Verification items for the finished model (mm, model axes). A direction names the side the tool comes from. Round coordinates to 2 decimals unless told otherwise and drop trailing zeros. Order: outer loops, then holes, each group sorted by start corner. A loop starts at its lowest first (then second) coordinate and runs counter-clockwise, first axis right, second up. Notation, with made-up numbers: (4.5, -17) -> (23.5, -17) arc R23 ccw to (23.5, 5) -> close; hole circle Ø6 at (60, 36.5). An arc over 180 degrees is marked (long way). Return JSON: item names as keys, results as strings. Group by question number.
Item 1: Sectioned sample at A-A on y = -3.75. Record the cut outline in (x, z).
Item 2: Draft check along Z on faces 3 (the flat face through (348.1, -10.94, 0.17)), 4 (the flat face through (174, -12.5, 0)), 5 (the flat face through (174, 10.5, 0)). Enter one of: pulls with the +Z half, pulls with the -Z half, needs draft (parallel to the pull), parting line crosses it, or undercut.
Item 3: Sectioned sample at B-B on z = -6.75. Record the cut outline in (x, y), plus the area to 3 significant figures.
Item 4: Sectioned sample at C-C on x = 159.5. Record the cut outline in (y, z).
Item 5: Scan lines: probe 1 along Y at (x, z) = (208, 2.25); probe 2 along X at (y, z) = (-10.75, -4.25). Record each from-to range of solid material in increasing order. Write a range as from..to.
Item 6: Access from +Z, -Z, +X, -X, +Y, -Y to the whole of each face (thin tool, end or side, straight path). Record for faces 1 (the flat face through (174, 0, 10.5)), 2 (the flat face through (174, 0, -12.5)).
```python
from build123d import *

# Parameters (mm, degrees)
F0_W        = 25
F0_H        = 25
F0_W_2      = 21
F0_H_2      = 21
F1_DEPTH    = 353.347
F2_T1_DEPTH = 154.6335196453
F3_T1_DEPTH = 154.6335196453


# Not quite as in the source:
# - a fillet or chamfer that OpenCascade refuses, or shapes differently, is made with other operations: its cross-section is extruded or revolved along the edge and cut away or added


with BuildPart() as f1:
    # F0 (on Right) → F1 (new body)
    with BuildSketch(Plane.YZ):
        Rectangle(F0_W, F0_H)
        Rectangle(F0_W_2, F0_H_2, mode=Mode.SUBTRACT)
    extrude(amount=F1_DEPTH)

    # F2: chamfer of 25 x 10.3553390593 on 1 edges, made by hand

    # F2_s2 → F2_t1 (cut)
    with BuildSketch(Plane.XZ.offset(-77.3167598227)):
        Polygon((342.9916609407, 12.5), (353.347, -12.5), (353.347, 12.5), align=None)
    extrude(amount=F2_T1_DEPTH, mode=Mode.SUBTRACT)

    # F3: chamfer of 25 x 10.3553390593 on 1 edges, made by hand

    # F3_s2 → F3_t1 (cut)
    with BuildSketch(Plane.XZ.offset(-77.3167598227)):
        Polygon((0, -12.5), (10.3553390593, 12.5), (0, 12.5), align=None)
    extrude(amount=F3_T1_DEPTH, mode=Mode.SUBTRACT)


solid = f1.part
```
Recorded:
{
 "1": {"outline": "(0, -12.5) -> (353.35, -12.5) -> (352.52, -10.5) -> (0.83, -10.5) -> close; (9.53, 10.5) -> (343.82, 10.5) -> (342.99, 12.5) -> (10.36, 12.5) -> close"},
 "2": {"face 3": "pulls with the +Z half", "face 4": "needs draft", "face 5": "undercut"},
 "3": {"outline": "(2.38, -12.5) -> (350.97, -12.5) -> (350.97, -10.5) -> (2.38, -10.5) -> close; (2.38, 10.5) -> (350.97, 10.5) -> (350.97, 12.5) -> (2.38, 12.5) -> close", "area": "1,390 mm²"},
 "4": {"outline": "(-12.5, -12.5) -> (12.5, -12.5) -> (12.5, 12.5) -> (-12.5, 12.5) -> close; hole (-10.5, -10.5) -> (10.5, -10.5) -> (10.5, 10.5) -> (-10.5, 10.5) -> close"},
 "5": {"probe 1": "-12.5..-10.5, 10.5..12.5", "probe 2": "3.42..349.93"},
 "6": {"face 1": "+X, -X", "face 2": "-Z, +X, -X, +Y, -Y"}
}
